```python
from build123d import *

# Parameters (mm, degrees)
SKETCH1_W           = 20
SKETCH1_H           = 20
BOSS_EXTRUDE1_DEPTH = 40
CUT_EXTRUDE1_DEPTH  = 46.82575695
FILLET1_R           = 1


with BuildPart() as part:
    # Sketch1 → Boss-Extrude1 (new body)
    with BuildSketch(Plane(origin=(0, 0, 0), x_dir=(1, 0, 0), z_dir=(0, 1, 0))):
        Rectangle(SKETCH1_W, SKETCH1_H)
    extrude(amount=BOSS_EXTRUDE1_DEPTH)

    # Sketch2 → Cut-Extrude1 (cut, through all)
    with BuildSketch(Plane.XY.offset(10)):
        Polygon((-10, 20), (10, 40), (-10, 40), align=None)
        Polygon((10, 0), (-10, 20), (-10, 0), align=None)
    extrude(amount=-CUT_EXTRUDE1_DEPTH, mode=Mode.SUBTRACT)

    # Fillet1
    fillet1_edges = [part.edges().sort_by_distance(p)[0] for p in [
        (0, 30, 10),
        (0, 30, -10),
        (0, 10, 10),
        (0, 10, -10),
        (10, 20, 10),
        (10, 20, -10),
    ]]
    fillet(fillet1_edges, radius=FILLET1_R)


solid = part.part
```
Design review of the part built by this model. Coordinates are the model's own, in mm. Round coordinates to 2 decimals unless told otherwise and drop trailing zeros. Order: outer loops, then holes, each group sorted by start corner. A loop starts at its lowest first (then second) coordinate and runs counter-clockwise, first axis right, second up. Notation, with made-up numbers: M 50,-23.75 L 89,-23.75 A31 cw 89,6.25 Z; hole C 82,-7 d7. An arc over 180 degrees is marked long. Put each result on its own line as item: value.
Q1. Insertion check: pin 1 Ø10 at (y, z) = (5.5, -4.5) entering from -X; pin 2 Ø4 at (x, y) = (2.5, 5) entering from +Z; pin 3 Ø8 at (x, z) = (-8, -5) entering from -Y. Each pin has a flat end and moves straight along its axis. Give the tip position at first contact, or say it passes through.
Reported:
pin 1: x = -0.5
pin 2: z = 9.64
pin 3: y = 14
Q2. Consider section A-A (z = 3). State the section outline as (x, y) points, and give its area (3 significant figures).
Reported:
outline: M -10,20 L 10,0 L 10,40 Z
area: 400 mm²
Q3. To check wall thickness, follow line 1 (X direction, y = 8.5, z = -3); line 2 (X direction, y = 21, z = -0.5); line 3 (Z direction, x = 6.25, y = 4.5). State the ranges of each line that lie inside material, in increasing order.
Reported:
line 1: 1.5 to 10
line 2: -9 to 10
line 3: -9.88 to 9.88
